from build123d import *

# Parameters (mm, degrees)
SKETCH1_W           = 120
SKETCH1_H           = 60
BOSS_EXTRUDE1_DEPTH = 2
CHAMFER2_SIZE       = 10
SKETCH2_W           = 38.34314575
SKETCH2_H           = 2
BOSS_EXTRUDE2_DEPTH = 15
FILLET1_R           = 2
SKETCH4_R           = 2.5
SKETCH4_R_2         = 1
BOSS_EXTRUDE3_DEPTH = 4
SKETCH6_W           = 61
SKETCH6_H           = 14.6
BOSS_EXTRUDE5_DEPTH = 15
CUT_EXTRUDE2_START  = -3
CUT_EXTRUDE2_DEPTH  = 55
CHAMFER3_SIZE       = 4
SKETCH9_W           = 14
SKETCH9_H           = 16
SKETCH9_W_2         = 10
SKETCH9_H_2         = 12
BOSS_EXTRUDE6_DEPTH = 4
SKETCH10_R          = 3
SKETCH10_R_2        = 1.5
BOSS_EXTRUDE8_DEPTH = 4
BOSS_EXTRUDE9_START = 10
SKETCH12_R          = 3
SKETCH12_R_2        = 1.8
BOSS_EXTRUDE9_DEPTH = 10
CHAMFER4_SIZE       = 2
SKETCH13_W          = 142.36375675
SKETCH13_H          = 36.547684865
CUT_EXTRUDE3_DEPTH  = 85
CUT_EXTRUDE4_START  = -4
CUT_EXTRUDE4_DEPTH  = 2


with BuildPart() as part:
    # Sketch1 → Boss-Extrude1 (new body)
    with BuildSketch(Plane.XY):
        with Locations((60, 30)):
            Rectangle(SKETCH1_W, SKETCH1_H)
    extrude(amount=BOSS_EXTRUDE1_DEPTH)

    # Chamfer2
    chamfer2_edges = [part.edges().sort_by_distance(p)[0] for p in [
        (0, 60, 1),
        (120, 60, 1),
        (120, 0, 1),
        (0, 0, 1),
    ]]
    chamfer(chamfer2_edges, length=CHAMFER2_SIZE)

    # Sketch2 → Boss-Extrude2 (add)
    with BuildSketch(Plane.XY.offset(2)):
        Polygon((10.828427125, 2), (109.171572875, 2), (118, 10.828427125), (118, 49.171572875), (109.171572875, 58), (109.171572875, 60), (110, 60), (120, 50), (120, 10), (110, 0), (10, 0), (0, 10), (0, 50), (10, 60), (10.828427125, 60), (10.828427125, 58), (2, 49.171572875), (2, 10.828427125), align=None)
        with Locations((60, 59)):
            Rectangle(SKETCH2_W, SKETCH2_H)
    extrude(amount=BOSS_EXTRUDE2_DEPTH)

    # Fillet1
    fillet1_edges = [part.edges().sort_by_distance(p)[0] for p in [
        (113.585786438, 53.585786438, 2),
        (118, 30, 2),
        (113.585786438, 6.414213562, 2),
        (60, 2, 2),
        (6.414213562, 6.414213562, 2),
        (2, 30, 2),
        (6.414213562, 53.585786438, 2),
        (60, 58, 2),
    ]]
    fillet(fillet1_edges, radius=FILLET1_R)

    # Sketch4 → Boss-Extrude3 (add)
    with BuildSketch(Plane.XY.offset(2)):
        with Locations((33, 41)):
            Circle(SKETCH4_R)
        with Locations((33, 41)):
            Circle(SKETCH4_R_2, mode=Mode.SUBTRACT)
    extrude(amount=BOSS_EXTRUDE3_DEPTH)

    # Sketch6 → Boss-Extrude5 (add)
    with BuildSketch(Plane.XY.offset(2)):
        with Locations((60, 9.3)):
            Rectangle(SKETCH6_W, SKETCH6_H)
    extrude(amount=BOSS_EXTRUDE5_DEPTH)

    # Sketch7 → Cut-Extrude2 (cut)
    with BuildSketch(Plane.ZY.offset(-29.5).offset(CUT_EXTRUDE2_START)):
        with BuildLine():
            ThreePointArc((16.8, 9.3), (14.661879503, 14.461879503), (9.5, 16.6))
            Line((9.5, 16.6), (9.5, 2))
            ThreePointArc((9.5, 2), (14.661879503, 4.138120497), (16.8, 9.3))
        make_face()
        with BuildLine():
            Line((9.5, 2), (9.5, 16.6))
            ThreePointArc((9.5, 16.6), (2.2, 9.3), (9.5, 2))
        make_face()
        with BuildLine():
            Line((17, 16.6), (9.5, 16.6))
            ThreePointArc((9.5, 16.6), (14.661879503, 14.461879503), (16.8, 9.3))
            ThreePointArc((16.8, 9.3), (14.661879503, 4.138120497), (9.5, 2))
            Line((9.5, 2), (17, 2))
            Line((17, 2), (17, 16.6))
        make_face()
    extrude(amount=-CUT_EXTRUDE2_DEPTH, mode=Mode.SUBTRACT)

    # Chamfer3
    chamfer3_edges = [part.edges().sort_by_distance(p)[0] for p in [
        (31, 16.6, 17),
        (89, 16.6, 17),
    ]]
    chamfer(chamfer3_edges, length=CHAMFER3_SIZE)

    # Sketch9 → Boss-Extrude6 (add)
    with BuildSketch(Plane.XY.offset(2)):
        with Locations((45, 41)):
            Rectangle(SKETCH9_W, SKETCH9_H)
        with Locations((45, 41)):
            Rectangle(SKETCH9_W_2, SKETCH9_H_2, mode=Mode.SUBTRACT)
    extrude(amount=BOSS_EXTRUDE6_DEPTH)

    # Sketch10 → Boss-Extrude8 (add)
    with BuildSketch(Plane.XY.offset(2)):
        with Locations((14.828427125, 57)):
            Circle(SKETCH10_R)
        with Locations((14.828427125, 57)):
            Circle(SKETCH10_R_2, mode=Mode.SUBTRACT)
        with Locations((105.171572875, 57)):
            Circle(SKETCH10_R)
        with Locations((105.171572875, 57)):
            Circle(SKETCH10_R_2, mode=Mode.SUBTRACT)
    extrude(amount=BOSS_EXTRUDE8_DEPTH)

    # Sketch13 → Cut-Extrude3 (cut)
    with BuildSketch(Plane(origin=(0, 60, 0), x_dir=(1, 0, 0), z_dir=(0, 1, 0))):
        with Locations((60.382698271, -6.82770274)):
            Rectangle(SKETCH13_W, SKETCH13_H)
    extrude(amount=-CUT_EXTRUDE3_DEPTH, mode=Mode.SUBTRACT)


with BuildPart() as body_2:
    # Sketch12 → Boss-Extrude9 (new body)
    with BuildSketch(Plane.XY.offset(17).offset(BOSS_EXTRUDE9_START)):
        with Locations((14.828427125, 57)):
            Circle(SKETCH12_R)
        with Locations((14.828427125, 57)):
            Circle(SKETCH12_R_2, mode=Mode.SUBTRACT)
        with BuildLine():
            Line((11.828427125, 63), (11.828427125, 57))
            ThreePointArc((11.828427125, 57), (14.828427125, 60), (17.828427125, 57))
            Line((17.828427125, 57), (17.828427125, 60))
            Line((17.828427125, 60), (42.76580882, 60))
            Line((42.76580882, 60), (42.76580882, 63))
            Line((42.76580882, 63), (11.828427125, 63))
        make_face()
    extrude(amount=BOSS_EXTRUDE9_DEPTH)

    # Chamfer4
    chamfer4_edges = [body_2.edges().sort_by_distance(p)[0] for p in [
        (11.828427125, 63, 32),
        (42.76580882, 63, 32),
        (17.828427125, 60, 32),
    ]]
    chamfer(chamfer4_edges, length=CHAMFER4_SIZE)

    # Sketch14 → Cut-Extrude4 (cut)
    with BuildSketch(Plane.XY.offset(37).offset(CUT_EXTRUDE4_START)):
        Polygon((32.828427125, 60), (32.828427125, 61.5), (17.828427125, 61.5), (17.828427125, 58), (28.911209964, 56.857462596), align=None)
    extrude(amount=-CUT_EXTRUDE4_DEPTH, mode=Mode.SUBTRACT)


solid = body_2.part
Geometry check sheet. Reference: the model listing, model coordinates, mm. A direction names the side the tool comes from. Round coordinates to 2 decimals unless told otherwise and drop trailing zeros. Write each loop counter-clockwise with the first axis right and the second up, starting at its lowest first coordinate (ties: lowest second). Pieces come first, ordered by that corner, then holes. Notation, with made-up numbers: (-34, -14) - (-8, -14) arc R12 ccw to (-8, -9) - close; hole circle Ø1 at (43, 59.5). An arc over 180 degrees is marked (long way). One line per item, written item: value.
1. Depth check by flat-ended pin: pin 1 Ø1.5 at (y, z) = (55.5, 35.5) entering from +X; pin 2 Ø0.6 at (x, z) = (24, 32.5) entering from -Y; pin 3 Ø5 at (y, z) = (56, 32.5) entering from +X. Enter the tip coordinate at first touch or a pass-through.
The answers:
pin 1: stops at x = 17.73
pin 2: stops at y = 61.5
pin 3: stops at x = 18.28
2. Cross-section at A-A on x = 30. Record the boundary of the cut face in (y, z), and give its area (3 significant figures).
The answers:
outline: (60, 27) - (63, 27) - (63, 37) - (60, 37) - (60, 33) - (61.5, 33) - (61.5, 31) - (60, 31) - close
area: 27.0 mm^2
3. Cross-section at D-D on x = 38. Record the boundary of the cut face in (y, z), and give its area (3 significant figures).
The answers:
outline: (60, 27) - (63, 27) - (63, 37) - (60, 37) - close
area: 30.0 mm^2
4. Set-up check for faces 4 (the face through (24, 61, 37)), 5 (the face through (31.1, 60, 30.8)), 6 (the face through (25, 61, 33)): record each of +Z, -Z, +X, -X, +Y, -Y from which the full face is reachable in a straight line by a thin tool's end or side.
The answers:
face 4: +Z, +X, -X, +Y, -Y
face 5: +Z, -Z, +X, -Y
face 6: -Y
5. Scan lines: L1, parallel to Z at x = 31.5, y = 60.5; L2, parallel to Y at x = 29, z = 33.25; L3, parallel to Y at x = 14, z = 32.25. Record each from-to range of solid material in increasing order.
The answers:
L1: z = 27 to 31, 33 to 37
L2: y = 60 to 63
L3: y = 54.12 to 55.4, 58.6 to 63
6. Mould release check, pull along X, two halves, no side actions. Record for faces 1 (the face through (41.752, 62.014, 31.93)), 2 (the face through (17.828, 58, 32)), 3 (the face through (24, 61, 27)): released by +X, released by -X, zero draft, split by the parting line, or undercut.
The answers:
face 1: released by +X
face 2: undercut
face 3: zero draft
7. Cross-section at B-B on z = 33.5. Record the boundary of the cut face in (x, y), and give its area (3 significant figures).
The answers:
outline: (11.83, 57) arc R3 ccw to (17.83, 57) - (17.83, 58) - (19.83, 60) - (42.77, 60) - (42.77, 61) - (40.77, 63) - (13.83, 63) - (11.83, 61) - close; hole circle Ø3.6 at (14.83, 57)
area: 113 mm^2
8. Cross-section at C-C on y = 59.25. Record the boundary of the cut face in (x, z), and give its area (3 significant figures).
The answers:
outline: (11.83, 27) - (19.08, 27) - (19.08, 31) - (17.83, 31) - (17.83, 33) - (19.08, 33) - (19.08, 37) - (11.83, 37) - close
area: 70.0 mm^2
